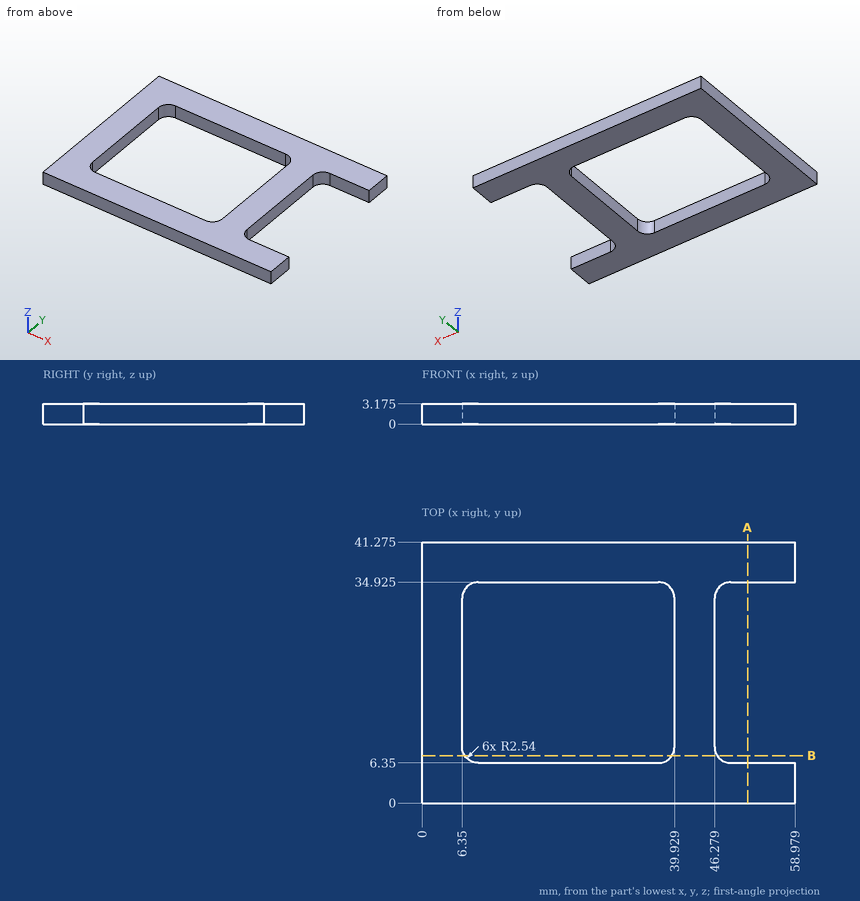
Can you work these out from the drawing? Everything is in mm from the part's minimum corner. Round coordinates to 2 decimals unless told otherwise and drop trailing zeros. Order: outer loops, then holes, each group sorted by start corner. A loop starts at its lowest first (then second) coordinate and runs counter-clockwise, first axis right, second up. Notation, with made-up numbers: (68.5, 8) - (72.5, 8) arc R29 ccw to (72.5, 33) - close; hole circle Ø1 at (65.25, 71.5). An arc over 180 degrees is marked (long way). Answer in a Markdown table with one row per item.
(1) Suppose I cut it at A-A, the plane x = 51.5. Please give me the cut outline in (y, z) (3 decimals), plus the area to 3 significant figures.
From the geometry:
| item | result |
|---|---|
| outline | (0, 0) - (6.35, 0) - (6.35, 3.175) - (0, 3.175) - close; (34.925, 0) - (41.275, 0) - (41.275, 3.175) - (34.925, 3.175) - close |
| area | 40.3 mm2 |
(2) Suppose I cut it at B-B, the plane y = 7.5. Please give me the cut outline in (x, z) (1 decimal).
From the geometry:
| item | result |
|---|---|
| outline | (0, 0) - (6.8, 0) - (6.8, 3.2) - (0, 3.2) - close; (39.5, 0) - (46.7, 0) - (46.7, 3.2) - (39.5, 3.2) - close |
(3) Please list where these lines run through material, in increasing order: L1, parallel to Y at x = 15, z = 0.5 (3 decimals); L2, parallel to X at y = 12.5, z = 0.9; L3, parallel to Y at x = 8, z = 2.55 (1 decimal). Write a range as from..to.
From the geometry:
| item | result |
|---|---|
| L1 | y = 0..6.35, 34.925..41.275 |
| L2 | x = 0..6.35, 39.93..46.28 |
| L3 | y = 0..6.5, 34.8..41.3 |
